```python
from build123d import *

# Parameters (mm, degrees)
SKETCH1_W               = 30
SKETCH1_H               = 28
BOSS_EXTRUDE1_DEPTH     = 20
SKETCH2_W               = 16
SKETCH2_H               = 14
CUT_EXTRUDE1_DEPTH      = 39.678159212
SKETCH3_W               = 30
SKETCH3_H               = 6
BOSS_EXTRUDE2_DEPTH     = 12
RIB11_REACH             = 46.452
SKETCH4_WALL_W          = 109.343531998
SKETCH4_WALL_H          = 6
MIRROR2_COPY_1_REACH    = 46.452
MIRROR2_COPY_1_SKETCH_W = 109.343531998
MIRROR2_COPY_1_SKETCH_H = 6
SKETCH6_R               = 1.5
CUT_EXTRUDE2_DEPTH      = 34.120990323
CHAMFER1_SIZE           = 2
CHAMFER2_SIZE           = 2


with BuildPart() as part:
    # Sketch1 → Boss-Extrude1 (new body)
    with BuildSketch(Plane(origin=(0, 0, 0), x_dir=(1, 0, 0), z_dir=(0, 1, 0))):
        Rectangle(SKETCH1_W, SKETCH1_H)
    extrude(amount=BOSS_EXTRUDE1_DEPTH)

    # Sketch2 → Cut-Extrude1 (cut, through all)
    with BuildSketch(Plane(origin=(15, 0, 0), x_dir=(0, 0, -1), z_dir=(1, 0, 0))):
        with Locations((0, 7)):
            Rectangle(SKETCH2_W, SKETCH2_H)
    extrude(amount=-CUT_EXTRUDE1_DEPTH, mode=Mode.SUBTRACT)

    # Sketch3 → Boss-Extrude2 (add)
    with BuildSketch(Plane.XY.offset(14)):
        with Locations((0, 3)):
            Rectangle(SKETCH3_W, SKETCH3_H)
    boss_extrude2 = extrude(amount=BOSS_EXTRUDE2_DEPTH)

    # Sketch4 wall → Rib11 (add, up to next)
    with BuildSketch(Plane(origin=(15, 13, 20), x_dir=(0, -0.759256602365, 0.650791373456), z_dir=(0, -0.650791373456, -0.759256602365)), mode=Mode.PRIVATE) as rib11_sk1:
        with Locations((0, 3)):
            Rectangle(SKETCH4_WALL_W, SKETCH4_WALL_H)
    rib11_tool1 = extrude(rib11_sk1.sketch, amount=RIB11_REACH, mode=Mode.PRIVATE) - part.part
    rib11 = rib11_tool1.solids().sort_by_distance((15, 13, 20))[0]
    add(rib11)

    # Mirror1: Rib11 across plane
    add(rib11.mirror(Plane(origin=(0, 0, 0), x_dir=(0, 0, 1), z_dir=(1, 0, 0))))

    # Mirror2: Boss-Extrude2, Rib11 across plane
    add(boss_extrude2.mirror(Plane.XY))
    add(rib11.mirror(Plane.XY))

    # Mirror2 copy 1 sketch → Mirror2 copy 1 (add, up to next)
    with BuildSketch(Plane(origin=(-15, 13, -20), x_dir=(0, -0.759256602365, -0.650791373456), z_dir=(0, -0.650791373456, 0.759256602365)), mode=Mode.PRIVATE) as mirror2_copy_1_sk1:
        with Locations((0, 3)):
            Rectangle(MIRROR2_COPY_1_SKETCH_W, MIRROR2_COPY_1_SKETCH_H)
    mirror2_copy_1_tool1 = extrude(mirror2_copy_1_sk1.sketch, amount=MIRROR2_COPY_1_REACH, mode=Mode.PRIVATE) - part.part
    add(mirror2_copy_1_tool1.solids().sort_by_distance((-15, 13, -20))[0])

    # Sketch6 → Cut-Extrude2 (cut, through all)
    with BuildSketch(Plane(origin=(0, 6, 0), x_dir=(1, 0, 0), z_dir=(0, 1, 0))):
        with Locations(Location((0, -20, 0), (0, 0, 270))):
            Circle(SKETCH6_R)
    cut_extrude2 = extrude(amount=-CUT_EXTRUDE2_DEPTH, mode=Mode.SUBTRACT)

    # Chamfer1
    chamfer1_edges = [part.edges().sort_by_distance(p)[0] for p in [
        (0, 6, 18.5),
    ]]
    chamfer(chamfer1_edges, length=CHAMFER1_SIZE)

    # Mirror7: Cut-Extrude2 across plane
    add(cut_extrude2.mirror(Plane.XY), mode=Mode.SUBTRACT)

    # Chamfer2
    chamfer2_edges = [part.edges().sort_by_distance(p)[0] for p in [
        (0, 6, -18.5),
    ]]
    chamfer(chamfer2_edges, length=CHAMFER2_SIZE)


solid = part.part
```
The model under review builds one solid part; all positions refer to its coordinate system, in mm. A direction names the side the tool comes from. Round coordinates to 2 decimals unless told otherwise and drop trailing zeros. Order: outer loops, then holes, each group sorted by start corner. A loop starts at its lowest first (then second) coordinate and runs counter-clockwise, first axis right, second up. Notation, with made-up numbers: (21, -32) -> (59, -32) arc R14 ccw to (59, -28) -> close; hole circle Ø3 at (5.25, 7). An arc over 180 degrees is marked (long way). Use a Markdown table: item, result.
Q1. Tool access review of faces 1 (the flat face through (0, 7, -8)), 2 (the flat face through (-9, 11, -18)), 3 (the flat face through (0, 13, 14)): name each direction out of +Z, -Z, +X, -X, +Y, -Y from which nothing blocks a thin tool from reaching the whole face with its end or side.
Values:
| item | result |
|---|---|
| face 1 | +X, -X, -Y |
| face 2 | -Z, +Y |
| face 3 | +Z, +Y |
Q2. We need section B-B on z = 20. Write out the cut boundary in (x, y).
Values:
| item | result |
|---|---|
| outline | (-15, 0) -> (-1.5, 0) -> (-1.5, 4) -> (-3.5, 6) -> (-9, 6) -> (-9, 13) -> (-15, 13) -> close; (1.5, 0) -> (15, 0) -> (15, 13) -> (9, 13) -> (9, 6) -> (3.5, 6) -> (1.5, 4) -> close |
Q3. We need section C-C on x = 11.25. Write out the cut boundary in (y, z).
Values:
| item | result |
|---|---|
| outline | (0, -26) -> (6, -26) -> (20, -14) -> (20, 14) -> (6, 26) -> (0, 26) -> (0, 8) -> (14, 8) -> (14, -8) -> (0, -8) -> close |
Q4. For line 1 (Z direction, x = 8.25, y = 3); line 2 (Z direction, x = -3, y = 10); line 3 (X direction, y = 2.35, z = -20), list the stretches that pass through material, from the lowest coordinate up.
Values:
| item | result |
|---|---|
| line 1 | z = -26 to -8, 8 to 26 |
| line 2 | z = -14 to -8, 8 to 14 |
| line 3 | x = -15 to -1.5, 1.5 to 15 |
Q5. We need section A-A on x = 0. Write out the cut boundary in (y, z).
Values:
| item | result |
|---|---|
| outline | (0, -26) -> (6, -26) -> (6, -23.5) -> (4, -21.5) -> (0, -21.5) -> close; (0, -18.5) -> (4, -18.5) -> (6, -16.5) -> (6, -14) -> (20, -14) -> (20, 14) -> (6, 14) -> (6, 16.5) -> (4, 18.5) -> (0, 18.5) -> (0, 8) -> (14, 8) -> (14, -8) -> (0, -8) -> close; (0, 21.5) -> (4, 21.5) -> (6, 23.5) -> (6, 26) -> (0, 26) -> close |
Q6. We need section D-D on y = 11.75. Write out the cut boundary in (x, z).
Values:
| item | result |
|---|---|
| outline | (-15, -21.07) -> (-9, -21.07) -> (-9, -14) -> (9, -14) -> (9, -21.07) -> (15, -21.07) -> (15, -8) -> (-15, -8) -> close; (-15, 8) -> (15, 8) -> (15, 21.07) -> (9, 21.07) -> (9, 14) -> (-9, 14) -> (-9, 21.07) -> (-15, 21.07) -> close |
Q7. Clearance check with flat-ended pins moving along their axes: P1, Ø12, axis at x = 10.5, z = -19.5, coming from the -Y side; P2, Ø5, axis at x = 0.5, z = 0, coming from the -Y side; P3, Ø1, axis at x = 0.5, y = 13, coming from the -Z side; P4, Ø9.5, axis at x = 0, z = 20, coming from the +Y side. State where each tip first meets the part, or that it passes through.
Values:
| item | result |
|---|---|
| P1 | stops at y = 0 |
| P2 | stops at y = 14 |
| P3 | stops at z = -14 |
| P4 | stops at y = 6 |
Q8. Mouldability with a two-part tool opening along Z and no side actions: class faces 4 (the flat face through (-12, 13, -20)), 5 (the cylindrical face through (0.07, 2.03, 18.5)), 6 (the flat face through (-15, 14.2, -3.5)), 7 (the flat face through (0, 3, 26)) as +Z half, -Z half, draft (parallel to the pull), parting line (faces both ways), or undercut.
Values:
| item | result |
|---|---|
| face 4 | -Z half |
| face 5 | undercut |
| face 6 | draft |
| face 7 | +Z half |
